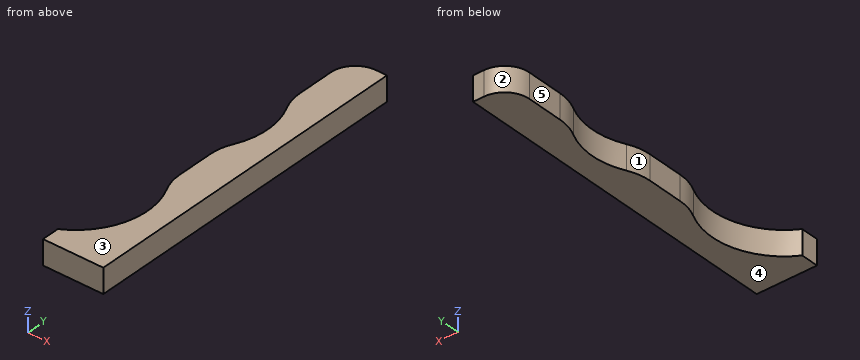
from build123d import *

# Parameters (mm, degrees)
BOSS_EXTRUDE1_DEPTH = 3.175


with BuildPart() as part:
    # Sketch1 → Boss-Extrude1 (new body)
    with BuildSketch(Plane.XY):
        with BuildLine():
            Line((3170.215202539, 2687.561172968), (3170.215202539, 2643.831916187))
            Line((3170.215202539, 2643.831916187), (3162.437951858, 2643.831916187))
            Line((3162.437951858, 2643.831916187), (3162.437951858, 2646.105339002))
            ThreePointArc((3162.437951858, 2646.105339002), (3166.805815961, 2651.440206281), (3166.271377044, 2658.314318641))
            ThreePointArc((3166.271377044, 2658.314318641), (3165.779748802, 2659.68421749), (3165.612951858, 2661.130073625))
            Line((3165.612951858, 2661.130073625), (3165.612951858, 2665.797353633))
            ThreePointArc((3165.612951858, 2665.797353633), (3165.779748802, 2667.243209769), (3166.271377044, 2668.613108618))
            ThreePointArc((3166.271377044, 2668.613108618), (3167.230702539, 2672.715663629), (3166.271377044, 2676.818218641))
            ThreePointArc((3166.271377044, 2676.818218641), (3165.779748802, 2678.18811749), (3165.612951858, 2679.633973625))
            Line((3165.612951858, 2679.633973625), (3165.612951858, 2684.386172968))
            ThreePointArc((3165.612951858, 2684.386172968), (3166.542887828, 2686.631236998), (3168.787951858, 2687.561172968))
            Line((3168.787951858, 2687.561172968), (3170.215202539, 2687.561172968))
        make_face()
    extrude(amount=BOSS_EXTRUDE1_DEPTH)


solid = part.part
Input: part model. Units: mm. Frame: model coordinates. Face numbers are marked on the shaded views. A direction names the side the tool comes from. Coordinates: 2 decimals unless noted, no trailing zeros. Loops run counter-clockwise (first coordinate to the right, second up) from the corner with the lowest first, then second, coordinate; pieces in that order, holes last.
Q1. Cut plane B-B (y = 2667). Output: boundary loops of the cut face in (x, z) (3 decimals), then the cut area to 3 significant figures.
Q2. Cut plane A-A (z = 2.3). Output: boundary loops of the cut face in (x, y) (3 decimals), then the cut area to 3 significant figures.
Q3. Material intervals for line 1 (Y direction, x = 3166.5, z = 2.2); line 2 (X direction, y = 2683, z = 1.2); line 3 (Y direction, x = 3165, z = 1.65), sorted ascending.
Q4. Contact query for flat-ended pins moving along their axis: pin 1 (1.6 mm diameter, centred on y = 2681, z = 2.5, fed in from -X); pin 2 (1 mm diameter, centred on x = 3166.5, z = 1, fed in from +Y). Output: stop coordinate, or through.
Q5. Draft query along Y for the marked faces 1, 2 and 3. Return one class per face: +Y half, -Y half, draft (parallel to the pull), parting line (faces both ways), or undercut.
Q6. Set-up query: the marked faces 4 and 5. Return all of +Z, -Z, +X, -X, +Y, -Y with unobstructed straight access to the full face (end or side cutting, diameter ignored); none if empty.
Q7. Cut plane C-C (x = 3164.5). Output: boundary loops of the cut face in (y, z) (3 decimals), then the cut area to 3 significant figures.
Working result:
1. outline: (3165.728, 0) - (3170.215, 0) - (3170.215, 3.175) - (3165.728, 3.175) - close
1. area: 14.2 mm2
2. outline: (3162.438, 2643.832) - (3170.215, 2643.832) - (3170.215, 2687.561) - (3168.788, 2687.561) arc R3.175 ccw to (3165.613, 2684.386) - (3165.613, 2679.634) arc R6.35 ccw to (3166.271, 2676.818) arc R9.252 cw to (3166.271, 2668.613) arc R6.35 ccw to (3165.613, 2665.797) - (3165.613, 2661.13) arc R6.35 ccw to (3166.271, 2658.314) arc R9.252 cw to (3162.438, 2646.105) - close
2. area: 187 mm2
3. line 1: y = 2643.83 to 2650.61, 2657.82 to 2669.11, 2676.32 to 2686.59
3. line 2: x = 3165.61 to 3170.22
3. line 3: y = 2643.83 to 2648.19
4. pin 1: stops at x = 3165.61
4. pin 2: stops at y = 2687.01
5. face 1: undercut
5. face 2: +Y half
5. face 3: draft
6. face 4: -Z, +X, -X, +Y, -Y
6. face 5: +Z, -Z, -X, +Y
7. outline: (2643.832, 0) - (2647.649, 0) - (2647.649, 3.175) - (2643.832, 3.175) - close
7. area: 12.1 mm2
